```python
from build123d import *

# Parameters (mm, degrees)
EXTRUDE_1_DEPTH      = 2
CUT_EXTRUDE_1_DEPTH  = 2
EXTRUDE_2_DEPTH      = 2
SKETCH_6_W           = 3.3
SKETCH_6_H           = 13
CUT_EXTRUDE_3_DEPTH  = 2
SKETCH_7_W           = 6
SKETCH_7_H           = 5
CUT_EXTRUDE_4_DEPTH  = 2
CUT_EXTRUDE_5_DEPTH  = 2
CUT_EXTRUDE_7_DEPTH  = 10
CUT_EXTRUDE_9_DEPTH  = 10
FILLET_1_R           = 5
CUT_EXTRUDE_10_DEPTH = 50
SKETCH_13_R          = 1.65
CUT_EXTRUDE_11_DEPTH = 50
FILLET_2_R           = 5
CUT_EXTRUDE_13_DEPTH = 50
FILLET_4_R           = 2
FILLET_5_R           = 3


with BuildPart() as part:
    # 草图1 → 凸台-拉伸1 (new body)
    with BuildSketch(Plane.XY):
        Polygon((-20, -65), (-35, -65), (-35, 65), (35, 65), (35, -65), (22, -65), (22, -68), (10, -68), (10, -65), (-8, -65), (-8, -68), (-20, -68), align=None)
    extrude(amount=EXTRUDE_1_DEPTH)

    # 草图2 → 切除-拉伸1 (cut)
    with BuildSketch(Plane.XY.offset(2)):
        Polygon((-35, -65), (-19.130571736, 25), (10.869428264, 65), (-35, 65), align=None)
    extrude(amount=-CUT_EXTRUDE_1_DEPTH, mode=Mode.SUBTRACT)

    # 草图3 → 凸台-拉伸2 (add)
    with BuildSketch(Plane.XY.offset(2)):
        Polygon((35, 65), (115, 65), (85, 0), (35, -65), align=None)
    extrude(amount=-EXTRUDE_2_DEPTH)

    # 草图6 → 切除-拉伸3 (cut)
    with BuildSketch(Plane.XY.offset(2)):
        with Locations((-25.2, -58.5)):
            Rectangle(SKETCH_6_W, SKETCH_6_H)
        with Locations((27.2, -58.5)):
            Rectangle(SKETCH_6_W, SKETCH_6_H)
    extrude(amount=-CUT_EXTRUDE_3_DEPTH, mode=Mode.SUBTRACT)

    # 草图7 → 切除-拉伸4 (cut)
    with BuildSketch(Plane.XY.offset(2)):
        with Locations((-25.2, -57)):
            Rectangle(SKETCH_7_W, SKETCH_7_H)
        with Locations((27.2, -57)):
            Rectangle(SKETCH_7_W, SKETCH_7_H)
    extrude(amount=-CUT_EXTRUDE_4_DEPTH, mode=Mode.SUBTRACT)

    # 草图8 → 切除-拉伸5 (cut)
    with BuildSketch(Plane.XY.offset(2)):
        Polygon((46.581829906, -49.943621123), (14.201899011, -4.308455167), (24.89214771, 30.117769456), (102.152743187, 37.164276905), (85, 0), align=None)
    extrude(amount=-CUT_EXTRUDE_5_DEPTH, mode=Mode.SUBTRACT)

    # 草图9 → 切除-拉伸7 (cut)
    with BuildSketch(Plane.XY.offset(2)):
        with BuildLine():
            Line((-12.8, 19.8), (-1.9, 19.8))
            ThreePointArc((-1.9, 19.8), (-0.8, 18.7), (0.3, 19.8))
            Line((0.3, 19.8), (0.3, 22.3))
            ThreePointArc((0.3, 22.3), (-0.8, 23.4), (-1.9, 22.3))
            Line((-1.9, 22.3), (-12.8, 22.3))
            ThreePointArc((-12.8, 22.3), (-13.9, 23.4), (-15, 22.3))
            Line((-15, 22.3), (-15, 19.8))
            ThreePointArc((-15, 19.8), (-13.9, 18.7), (-12.8, 19.8))
        make_face()
    extrude(amount=-CUT_EXTRUDE_7_DEPTH, mode=Mode.SUBTRACT)

    # 草图11 → 切除-拉伸9 (cut)
    with BuildSketch(Plane(origin=(0, 0, 0), x_dir=(-1, 0, 0), z_dir=(0, 0, -1))):
        Polygon((-2.431069725, -5), (-30.812630494, -45), (21.319194267, -45), (14.266115039, -5), align=None)
    extrude(amount=-CUT_EXTRUDE_9_DEPTH, mode=Mode.SUBTRACT)

    # 圆角1
    fillet_1_edges = [part.edges().sort_by_distance(p)[0] for p in [
        (46.581829906, -49.943621123, 1),
        (14.201899011, -4.308455167, 1),
        (24.89214771, 30.117769456, 1),
        (2.431069725, -5, 1),
        (-14.266115039, -5, 1),
        (-21.319194267, -45, 1),
        (30.812630494, -45, 1),
    ]]
    fillet(fillet_1_edges, radius=FILLET_1_R)

    # 草图12 → 切除-拉伸10 (cut)
    with BuildSketch(Plane.XY.offset(2)):
        with BuildLine():
            Line((22.2, 54.1), (33, 54.1))
            ThreePointArc((33, 54.1), (34.1, 55.2), (35.2, 54.1))
            Line((35.2, 54.1), (35.2, 51.6))
            ThreePointArc((35.2, 51.6), (34.1, 50.5), (33, 51.6))
            Line((33, 51.6), (22.2, 51.6))
            ThreePointArc((22.2, 51.6), (21.1, 50.5), (20, 51.6))
            Line((20, 51.6), (20, 54.1))
            ThreePointArc((20, 54.1), (21.1, 55.2), (22.2, 54.1))
        make_face()
        with BuildLine():
            Line((62.2, 51.6), (73, 51.6))
            ThreePointArc((73, 51.6), (74.1, 50.5), (75.2, 51.6))
            Line((75.2, 51.6), (75.2, 54.1))
            ThreePointArc((75.2, 54.1), (74.1, 55.2), (73, 54.1))
            Line((73, 54.1), (62.2, 54.1))
            ThreePointArc((62.2, 54.1), (61.1, 55.2), (60, 54.1))
            Line((60, 54.1), (60, 51.6))
            ThreePointArc((60, 51.6), (61.1, 50.5), (62.2, 51.6))
        make_face()
    extrude(amount=-CUT_EXTRUDE_10_DEPTH, mode=Mode.SUBTRACT)

    # 草图13 → 切除-拉伸11 (cut)
    with BuildSketch(Plane.XY.offset(2)):
        with Locations((9.1, 52.85)):
            Circle(SKETCH_13_R)
        with Locations((49.1, 52.85)):
            Circle(SKETCH_13_R)
        with Locations((95.1, 52.85)):
            Circle(SKETCH_13_R)
    extrude(amount=-CUT_EXTRUDE_11_DEPTH, mode=Mode.SUBTRACT)

    # 圆角2
    fillet_2_edges = [part.edges().sort_by_distance(p)[0] for p in [
        (102.152743187, 37.164276905, 1),
        (10.869428264, 65, 1),
        (-19.130571736, 25, 1),
    ]]
    fillet(fillet_2_edges, radius=FILLET_2_R)

    # 草图15 → 切除-拉伸13 (cut)
    with BuildSketch(Plane.XY.offset(2)):
        Polygon((6.869428264, 43), (-4.380571736, 28), (14.369428264, 28), (25.619428264, 43), align=None)
    extrude(amount=-CUT_EXTRUDE_13_DEPTH, mode=Mode.SUBTRACT)

    # 圆角4
    fillet_4_edges = [part.edges().sort_by_distance(p)[0] for p in [
        (6.869428264, 43, 1),
        (25.619428264, 43, 1),
        (14.369428264, 28, 1),
        (-4.380571736, 28, 1),
    ]]
    fillet(fillet_4_edges, radius=FILLET_4_R)

    # 圆角5
    fillet_5_edges = [part.edges().sort_by_distance(p)[0] for p in [
        (115, 65, 1),
    ]]
    fillet(fillet_5_edges, radius=FILLET_5_R)


solid = part.part
```
The model under review builds one solid part; all positions refer to its coordinate system, in mm. A direction names the side the tool comes from. Coordinates: 2 decimals unless noted, no trailing zeros. Write each loop counter-clockwise with the first axis right and the second up, starting at its lowest first coordinate (ties: lowest second). Pieces come first, ordered by that corner, then holes.
1) We need section D-D on x = 78. State the section outline as (y, z) points, then the cut area to 3 significant figures.
2) Clearance check with flat-ended pins moving along their axes: pin 1 Ø0.6 at (y, z) = (-53.5, 1) entering from -X; pin 2 Ø2 at (x, y) = (95.1, 52.85) entering from +Z; pin 3 Ø0.6 at (y, z) = (-66, 0.5) entering from -X; pin 4 Ø1 at (y, z) = (-53.5, 1) entering from -X. State where each tip first meets the part, or that it passes through.
3) To check wall thickness, follow probe 1 along Y at (x, z) = (27, 0.7); probe 2 along Y at (x, z) = (1.5, 1.55); probe 3 along X at (y, z) = (-54, 1.3). State the ranges of each line that lie inside material, in increasing order.
4) Machinability: for faces 1 (the face through (30.24, -26.91, 1.01)), 2 (the face through (25.61, -42.23, 1.01)), 3 (the face through (-27.28, -21.21, 1.01)), which of the approach directions +Z, -Z, +X, -X, +Y, -Y give a long, thin tool a straight path to every point of the face, cutting with its end or side? Answer none if there is none.
5) We need section A-A on x = 95.1. State the section outline as (y, z) points, then the cut area to 3 significant figures.
6) We need section B-B on z = 0.85. Count the separate pieces of the cut face and the enclosed holes in it, then the cut area to 3 significant figures.
7) The part is to be moulded in two halves that separate along Y. For faces 4 (the face through (112.86, 63.58, 0.99)), 5 (the face through (108.267, 50.411, 1.014)), 6 (the face through (48.885, 54.486, 1.014)), say which applies: pulls with the +Y half, pulls with the -Y half, needs draft (parallel to the pull), parting line crosses it, or undercut.
8) We need section C-C on x = 42.5. State the section outline as (y, z) points, then the cut area to 3 significant figures.
Answer list:
1. outline: (34.96, 0) - (65, 0) - (65, 2) - (34.96, 2) - close
1. area: 60.1 mm2
2. pin 1: stops at x = -33.03
2. pin 2: passes through
2. pin 3: stops at x = -20
2. pin 4: stops at x = -33.06
3. probe 1: y = -52 to -22.35, 30.15 to 51.6, 54.1 to 65
3. probe 2: y = -65 to -45, -5.28 to 28, 35.84 to 52.51
3. probe 3: x = -33.06 to -26.85, -23.55 to 25.55, 28.85 to 43.46
4. face 1: +Z, -Z, +X
4. face 2: +Z, -Z
4. face 3: +Z, -Z, -X, +Y
5. outline: (36.52, 0) - (51.2, 0) - (51.2, 2) - (36.52, 2) - close; (54.5, 0) - (65, 0) - (65, 2) - (54.5, 2) - close
5. area: 50.4 mm2
6. separate pieces: 1
6. enclosed holes: 8
6. area: 6,920 mm2
7. face 4: parting line crosses it
7. face 5: pulls with the -Y half
7. face 6: undercut
8. outline: (-55.25, 0) - (-44.19, 0) - (-44.19, 2) - (-55.25, 2) - close; (31.72, 0) - (65, 0) - (65, 2) - (31.72, 2) - close
8. area: 88.7 mm2
